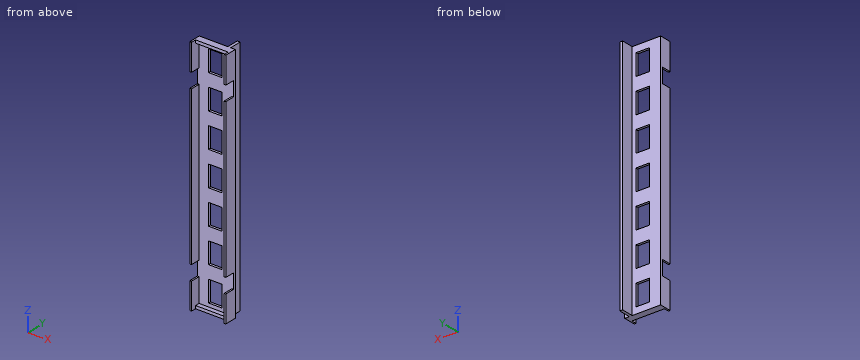
Autodesk Inventor part; units mm, degrees
ref_plane "p_XY" through (0, 0, 0) normal (0, 1, 0) x (1, 0, 0)
ref_plane "p_YZ" through (0, 0, 0) normal (1, 0, 0) x (0, 0, -1)
ref_plane "p_ZX" through (0, 0, 0) normal (0, 0, -1) x (0, 1, 0)
sketch "Sketch_1" plane through (0, 0, 0) normal (0, 0, 1) x (1, 0, 0)
  line L0 (-18.75, -12.5) -> (-17, -12.5)
  line L1 (-17, -12.5) -> (-17, -7.2)
  line L2 (-17, -7.2) -> (17, -7.2)
  line L3 (17, -7.2) -> (17, -12.5)
  line L4 (17, -12.5) -> (18.75, -12.5)
  line L5 (18.75, -12.5) -> (18.75, 0)
  line L6 (18.75, 0) -> (14, 0)
  line L7 (14, 0) -> (14, 12.5)
  line L8 (14, 12.5) -> (11, 12.5)
  line L9 (11, 12.5) -> (11, 0)
  line L10 (11, 0) -> (-18.75, 0)
  line L11 (-18.75, 0) -> (-18.75, -12.5)
extrude "Extrusion1" add sketch "Sketch_1" along normal blind 250
sketch "Sketch_2" plane through (-18.75, 0, 0) normal (0, 1, 0) x (0, 0, 1)
  line L0 (6.645, 11.65) -> (28.795, 11.65)
  line L1 (28.795, 11.65) -> (28.795, 25.85)
  line L2 (28.795, 25.85) -> (6.645, 25.85)
  line L3 (6.645, 25.85) -> (6.645, 11.65)
extrude "Extrusion2" cut sketch "Sketch_2" against normal blind 8
sketch "Sketch_3" plane through (-18.75, 0, 0) normal (0, 1, 0) x (0, 0, 1)
  line L0 (42.355, 25.85) -> (42.355, 11.65)
  line L1 (42.355, 11.65) -> (64.505, 11.65)
  line L2 (64.505, 11.65) -> (64.505, 25.85)
  line L3 (64.505, 25.85) -> (42.355, 25.85)
extrude "Extrusion3" cut sketch "Sketch_3" against normal blind 8
sketch "Sketch_4" plane through (-18.75, 0, 0) normal (0, 1, 0) x (0, 0, 1)
  line L0 (78.065, 11.65) -> (100.215, 11.65)
  line L1 (100.215, 11.65) -> (100.215, 25.85)
  line L2 (100.215, 25.85) -> (78.065, 25.85)
  line L3 (78.065, 25.85) -> (78.065, 11.65)
extrude "Extrusion4" cut sketch "Sketch_4" against normal blind 8
sketch "Sketch_5" plane through (-18.75, 0, 0) normal (0, 1, 0) x (0, 0, 1)
  line L0 (113.775, 25.85) -> (113.775, 11.65)
  line L1 (113.775, 11.65) -> (135.925, 11.65)
  line L2 (135.925, 11.65) -> (135.925, 25.85)
  line L3 (135.925, 25.85) -> (113.775, 25.85)
extrude "Extrusion5" cut sketch "Sketch_5" against normal blind 8
sketch "Sketch_6" plane through (-18.75, 0, 0) normal (0, 1, 0) x (0, 0, 1)
  line L0 (149.485, 25.85) -> (149.485, 11.65)
  line L1 (149.485, 11.65) -> (171.635, 11.65)
  line L2 (171.635, 11.65) -> (171.635, 25.85)
  line L3 (171.635, 25.85) -> (149.485, 25.85)
extrude "Extrusion6" cut sketch "Sketch_6" against normal blind 8
sketch "Sketch_7" plane through (-18.75, 0, 0) normal (0, 1, 0) x (0, 0, 1)
  line L0 (185.195, 11.65) -> (207.345, 11.65)
  line L1 (207.345, 11.65) -> (207.345, 25.85)
  line L2 (207.345, 25.85) -> (185.195, 25.85)
  line L3 (185.195, 25.85) -> (185.195, 11.65)
extrude "Extrusion7" cut sketch "Sketch_7" against normal blind 8
sketch "Sketch_8" plane through (-18.75, 0, 0) normal (0, 1, 0) x (0, 0, 1)
  line L0 (220.905, 25.85) -> (220.905, 11.65)
  line L1 (220.905, 11.65) -> (243.055, 11.65)
  line L2 (243.055, 11.65) -> (243.055, 25.85)
  line L3 (243.055, 25.85) -> (220.905, 25.85)
extrude "Extrusion8" cut sketch "Sketch_8" against normal blind 8
sketch "Sketch_10" plane through (-18.75, -12.5, 0) normal (-1, 0, 0) x (0, 0, 1)
  line L0 (27.9, 10) -> (27.9, 0)
  line L1 (27.9, 0) -> (43.3, 0)
  line L2 (43.3, 0) -> (43.3, 10)
  line L3 (43.3, 10) -> (27.9, 10)
extrude "Extrusion9" cut sketch "Sketch_10" against normal blind 37.5
sketch "Sketch_11" plane through (-18.75, -12.5, 0) normal (-1, 0, 0) x (0, 0, 1)
  line L0 (206.7, 10) -> (206.7, 0)
  line L1 (206.7, 0) -> (222.1, 0)
  line L2 (222.1, 0) -> (222.1, 10)
  line L3 (222.1, 10) -> (206.7, 10)
extrude "Extrusion10" cut sketch "Sketch_11" against normal blind 37.5
sketch "Sketch_13" plane through (-17, -7.2, 0) normal (0, -1, 0) x (1, 0, 0)
  line L0 (0, 247) -> (0, 3)
  line L1 (0, 3) -> (34, 3)
  line L2 (34, 3) -> (34, 247)
  line L3 (34, 247) -> (0, 247)
extrude "Extrusion11" cut sketch "Sketch_13" against normal blind 4.7
ref_plane "p_XY" through (0, 0, 0) normal (0, 1, 0) x (1, 0, 0)
ref_plane "p_YZ" through (0, 0, 0) normal (1, 0, 0) x (0, 0, -1)
ref_plane "p_ZX" through (0, 0, 0) normal (0, 0, -1) x (0, 1, 0)
ref_plane "p1_XY" through (0, -9.5, 17.72) normal (1, 0, 0) x (0, 0, -1)
ref_plane "p1_YZ" through (0, -9.5, 17.72) normal (0, 0, -1) x (0, 1, 0)
ref_plane "p1_ZX" through (0, -9.5, 17.72) normal (0, 1, 0) x (1, 0, 0)
ref_plane "p2_XY" through (0, -9.5, 53.43) normal (1, 0, 0) x (0, 0, -1)
ref_plane "p2_YZ" through (0, -9.5, 53.43) normal (0, 0, -1) x (0, 1, 0)
ref_plane "p2_ZX" through (0, -9.5, 53.43) normal (0, 1, 0) x (1, 0, 0)
ref_plane "p3_XY" through (0, -9.5, 89.14) normal (1, 0, 0) x (0, 0, -1)
ref_plane "p3_YZ" through (0, -9.5, 89.14) normal (0, 0, -1) x (0, 1, 0)
ref_plane "p3_ZX" through (0, -9.5, 89.14) normal (0, 1, 0) x (1, 0, 0)
ref_plane "p4_XY" through (0, -9.5, 124.85) normal (1, 0, 0) x (0, 0, -1)
ref_plane "p4_YZ" through (0, -9.5, 124.85) normal (0, 0, -1) x (0, 1, 0)
ref_plane "p4_ZX" through (0, -9.5, 124.85) normal (0, 1, 0) x (1, 0, 0)
ref_plane "p5_XY" through (0, -9.5, 160.56) normal (1, 0, 0) x (0, 0, -1)
ref_plane "p5_YZ" through (0, -9.5, 160.56) normal (0, 0, -1) x (0, 1, 0)
ref_plane "p5_ZX" through (0, -9.5, 160.56) normal (0, 1, 0) x (1, 0, 0)
ref_plane "p6_XY" through (0, -9.5, 196.27) normal (1, 0, 0) x (0, 0, -1)
ref_plane "p6_YZ" through (0, -9.5, 196.27) normal (0, 0, -1) x (0, 1, 0)
ref_plane "p6_ZX" through (0, -9.5, 196.27) normal (0, 1, 0) x (1, 0, 0)
ref_plane "p7_XY" through (0, -9.5, 231.98) normal (1, 0, 0) x (0, 0, -1)
ref_plane "p7_YZ" through (0, -9.5, 231.98) normal (0, 0, -1) x (0, 1, 0)
ref_plane "p7_ZX" through (0, -9.5, 231.98) normal (0, 1, 0) x (1, 0, 0)
properties part number "PRO10282 Rollenleiste Abdeckung mit Seitenfuehrung 250"
Can you work these out from the model? Positions are in its coordinate system, mm. Round coordinates to 2 decimals unless told otherwise and drop trailing zeros. Loops run counter-clockwise (first coordinate to the right, second up) from the corner with the lowest first, then second, coordinate; pieces in that order, holes last. Notation, with made-up numbers: (-34, 40) -> (22, 40) arc R15 cw to (22, 63) -> close; hole circle Ø7 at (-39, -5.75). An arc over 180 degrees is marked (long way). One line per item, written item: value. Start each with the question number.
1. If we section it at B-B, the plane z = 118: Write out the boundary of the cut face in (x, y).
2. If we section it at D-D, the plane x = 2: Give the number of separate pieces and of enclosed holes in the cut face, then the cut area to 3 significant figures.
3. For pin 1 (2 mm diameter, centred on x = -0.5, y = -0.5, fed in from -Z); pin 2 (1 mm diameter, centred on x = -5, z = 209.5, fed in from +Y); pin 3 (3 mm diameter, centred on x = -12.5, z = 90.5, fed in from -Y); pin 4 (1.5 mm diameter, centred on x = 0, z = 248.5, fed in from -Y), each with a flat end and sliding along its axis, tell me the tip position at first contact or that it passes through.
4. If I drill on probe 1 along X at (y, z) = (-2.25, 157.5); probe 2 along X at (y, z) = (-7.75, 205); probe 3 along Y at (x, z) = (10, 52), over which ranges is the centre line in solid material (lowest first)?
5. If we section it at A-A, the plane y = -9.25: Write out the boundary of the cut face in (x, z).
6. If we section it at C-C, the plane z = 67: Write out the boundary of the cut face in (x, y).
Calculated:
1. outline: (-18.75, -12.5) -> (-17, -12.5) -> (-17, -2.5) -> (-7.1, -2.5) -> (-7.1, 0) -> (-18.75, 0) -> close; (7.1, -2.5) -> (17, -2.5) -> (17, -12.5) -> (18.75, -12.5) -> (18.75, 0) -> (14, 0) -> (14, 12.5) -> (11, 12.5) -> (11, 0) -> (7.1, 0) -> close
2. separate pieces: 8
2. enclosed holes: 0
2. area: 266 mm²
3. pin 1: stops at z = 0
3. pin 2: stops at y = 0
3. pin 3: stops at y = -2.5
3. pin 4: stops at y = -7.2
4. probe 1: x = -18.75 to -7.1, 7.1 to 18.75
4. probe 2: x = -18.75 to -17, 17 to 18.75
4. probe 3: y = -2.5 to 0
5. outline: (-18.75, 0) -> (-17, 0) -> (-17, 27.9) -> (-18.75, 27.9) -> close; (-18.75, 43.3) -> (-17, 43.3) -> (-17, 206.7) -> (-18.75, 206.7) -> close; (-18.75, 222.1) -> (-17, 222.1) -> (-17, 250) -> (-18.75, 250) -> close; (17, 0) -> (18.75, 0) -> (18.75, 27.9) -> (17, 27.9) -> close; (17, 43.3) -> (18.75, 43.3) -> (18.75, 206.7) -> (17, 206.7) -> close; (17, 222.1) -> (18.75, 222.1) -> (18.75, 250) -> (17, 250) -> close
6. outline: (-18.75, -12.5) -> (-17, -12.5) -> (-17, -2.5) -> (17, -2.5) -> (17, -12.5) -> (18.75, -12.5) -> (18.75, 0) -> (14, 0) -> (14, 12.5) -> (11, 12.5) -> (11, 0) -> (-18.75, 0) -> close
